Geometry: final body of the model. Coordinates: model frame, mm. A direction names the side the tool comes from. Give positions to 0.01 mm unless a question says otherwise; leave off trailing zeros. Loops run counter-clockwise (first coordinate to the right, second up) from the corner with the lowest first, then second, coordinate; pieces in that order, holes last. Notation, with made-up numbers: M -15.5,49 L 30.5,49 A12 ccw 30.5,54 Z; hole C -24.5,63.5 d4. An arc over 180 degrees is marked long. Put each result on its own line as item: value.
```python
from build123d import *

# Parameters (mm, degrees)
F0_W     = 550
F0_H     = 550
F1_DEPTH = 450
F3_DEPTH = 350


with BuildPart() as f1:
    # F0 (on Top) → F1 (new body)
    with BuildSketch(Plane.XY):
        with Locations((275, 275)):
            Rectangle(F0_W, F0_H)
    extrude(amount=-F1_DEPTH)

    # F2 (on face) → F3 (cut)
    with BuildSketch(Plane(origin=(0, 0, -450), x_dir=(1, 0, 0), z_dir=(0, 0, -1))):
        Polygon((450, 0), (100, 0), (100, -100), (0, -100), (0, -450), (100, -450), (100, -550), (450, -550), (450, -450), (550, -450), (550, -100), (450, -100), align=None)
    extrude(amount=-F3_DEPTH, mode=Mode.SUBTRACT)


solid = f1.part
```
Item 1: Pin query (flat end, axial travel): pin 1 Ø1 at (x, y) = (340.5, 411) entering from -Z; pin 2 Ø6 at (x, z) = (477, -92) entering from -Y. Return the tip coordinate at first contact, or that it passes through.
Output values:
pin 1: z = -100
pin 2: y = 0
Item 2: Section A-A on z = -362. Output: boundary loops of the cut face in (x, y), then the cut area to 3 significant figures.
Output values:
outline: M 0,0 L 100,0 L 100,100 L 0,100 Z; M 0,450 L 100,450 L 100,550 L 0,550 Z; M 450,0 L 550,0 L 550,100 L 450,100 Z; M 450,450 L 550,450 L 550,550 L 450,550 Z
area: 40,000 mm²
Item 3: Section D-D on x = 367. Output: boundary loops of the cut face in (y, z).
Output values:
outline: M 0,-100 L 550,-100 L 550,0 L 0,0 Z
Item 4: Line query: probe 1 along X at (y, z) = (464, -153); probe 2 along Z at (x, y) = (158.5, 176). Output: solid intervals per line, ascending. Write a range as [from, to].
Output values:
probe 1: [0, 100], [450, 550]
probe 2: [-100, 0]
Item 5: Mould query, pull axis X, two halves, no side actions, for faces 4 (the flat face through (0, 271, -72)), 5 (the flat face through (271, 279, 0)), 6 (the flat face through (271, 271, -100)). Classes: pulls with the +X half, pulls with the -X half, needs draft (parallel to the pull), parting line crosses it, or undercut.
Output values:
face 4: pulls with the -X half
face 5: needs draft
face 6: undercut
Item 6: Section B-B on x = 62. Output: boundary loops of the cut face in (y, z).
Output values:
outline: M 0,-450 L 100,-450 L 100,-100 L 450,-100 L 450,-450 L 550,-450 L 550,0 L 0,0 Z
Item 7: Set-up query: faces 1 (the flat face through (49, 450, -277)), 2 (the flat face through (49, 501, -450)), 3 (the flat face through (450, 501, -277)). Return all of +Z, -Z, +X, -X, +Y, -Y with unobstructed straight access to the full face (end or side cutting, diameter ignored); none if empty.
Output values:
face 1: -Z, +X, -X
face 2: -Z, +X, -X, +Y, -Y
face 3: -Z, +Y, -Y
